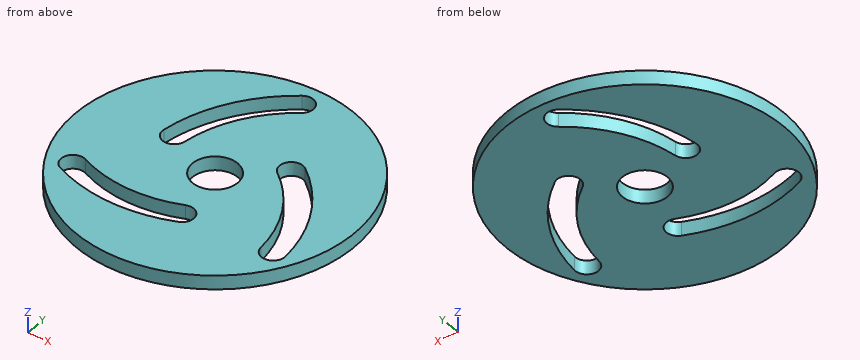
from build123d import *

# Parameters (mm, degrees)
SKETCH1_R           = 25
SKETCH1_R_2         = 4.064
BOSS_EXTRUDE1_DEPTH = 2.5


with BuildPart() as part:
    # Sketch1 → Boss-Extrude1 (new body)
    with BuildSketch(Plane.XY):
        with Locations((-21.594590832, 6.574444403)):
            Circle(SKETCH1_R)
        with Locations((-21.594590832, 6.574444403)):
            Circle(SKETCH1_R_2, mode=Mode.SUBTRACT)
        with BuildLine():
            ThreePointArc((-1.094322082, -3.289024862), (-4.554991799, 7.229910381), (-11.934322082, 15.486405892))
            ThreePointArc((-11.934322082, 15.486405892), (-14.870947643, 15.043426983), (-14.427968734, 12.106801422))
            ThreePointArc((-14.427968734, 12.106801422), (-8.192298494, 5.129910381), (-5.267968734, -3.758783976))
            ThreePointArc((-5.267968734, -3.758783976), (-2.946265851, -5.610727745), (-1.094322082, -3.289024862))
        make_face(mode=Mode.SUBTRACT)
        with BuildLine():
            ThreePointArc((-40.23766089, -6.093180307), (-29.39766089, -8.35562004), (-18.55766089, -6.093180307))
            ThreePointArc((-18.55766089, -6.093180307), (-17.472979098, -3.328498515), (-20.23766089, -2.243816723))
            ThreePointArc((-20.23766089, -2.243816723), (-29.39766089, -4.15562004), (-38.55766089, -2.243816723))
            ThreePointArc((-38.55766089, -2.243816723), (-41.322342681, -3.328498515), (-40.23766089, -6.093180307))
        make_face(mode=Mode.SUBTRACT)
        with BuildLine():
            ThreePointArc((-33.934461337, 10.432592457), (-32.082517568, 8.110889575), (-29.760814685, 9.962833344))
            ThreePointArc((-29.760814685, 9.962833344), (-26.836484925, 18.851527701), (-20.600814685, 25.828418741))
            ThreePointArc((-20.600814685, 25.828418741), (-20.157835776, 28.765044302), (-23.094461337, 29.208023212))
            ThreePointArc((-23.094461337, 29.208023212), (-30.473791621, 20.951527701), (-33.934461337, 10.432592457))
        make_face(mode=Mode.SUBTRACT)
    extrude(amount=BOSS_EXTRUDE1_DEPTH)


solid = part.part
Geometry check sheet. Reference: the model listing, model coordinates, mm. Give positions to 0.01 mm unless a question says otherwise; leave off trailing zeros. Loops run counter-clockwise (first coordinate to the right, second up) from the corner with the lowest first, then second, coordinate; pieces in that order, holes last.
(1) Section check B-B on y = 28. Record the cut outline in (x, z), then the cut area to 3 significant figures.
From the geometry:
outline: (-34.48, 0) - (-24.61, 0) - (-24.61, 2.5) - (-34.48, 2.5) - close; (-19.8, 0) - (-8.71, 0) - (-8.71, 2.5) - (-19.8, 2.5) - close
area: 52.4 mm2
(2) Section check C-C on x = -22. Record the cut outline in (y, z).
From the geometry:
outline: (-18.42, 0) - (-7.33, 0) - (-7.33, 2.5) - (-18.42, 2.5) - close; (-2.93, 0) - (2.53, 0) - (2.53, 2.5) - (-2.93, 2.5) - close; (10.62, 0) - (24.71, 0) - (24.71, 2.5) - (10.62, 2.5) - close; (29.61, 0) - (31.57, 0) - (31.57, 2.5) - (29.61, 2.5) - close
(3) Section check A-A on x = -29. Record the cut outline in (y, z).
From the geometry:
outline: (-17.3, 0) - (-8.35, 0) - (-8.35, 2.5) - (-17.3, 2.5) - close; (-4.15, 0) - (13.77, 0) - (13.77, 2.5) - (-4.15, 2.5) - close; (23.23, 0) - (30.45, 0) - (30.45, 2.5) - (23.23, 2.5) - close
(4) Section check D-D on y = 9. Record the cut outline in (x, z).
From the geometry:
outline: (-46.48, 0) - (-33.57, 0) - (-33.57, 2.5) - (-46.48, 2.5) - close; (-30.12, 0) - (-24.86, 0) - (-24.86, 2.5) - (-30.12, 2.5) - close; (-18.33, 0) - (-11, 0) - (-11, 2.5) - (-18.33, 2.5) - close; (-5.67, 0) - (3.29, 0) - (3.29, 2.5) - (-5.67, 2.5) - close
(5) Thickness scan on L1, parallel to Y at x = -30, z = 0.25; L2, parallel to Y at x = -24, z = 1.65; L3, parallel to Y at x = -20.5, z = 2.1. Record the ranges inside material, lowest first.
From the geometry:
L1: y = -16.97 to -8.35, -4.15 to 9.2, 21.74 to 30.12
L2: y = -18.31 to -7.81, -3.51 to 3.3, 9.85 to 22.75, 28.51 to 31.46
L3: y = -18.4 to -6.85, -2.36 to 2.66, 10.49 to 25.91, 29.13 to 31.55
